```python
from build123d import *

# Parameters (mm, degrees)
ESQUISSE1_W             = 20
ESQUISSE1_H             = 52
BOSS_EXTRU_1_DEPTH      = 3
ESQUISSE2_R             = 1.5
ENL_V_MAT_EXTRU_1_DEPTH = 3
ESQUISSE3_R             = 5
ENL_V_MAT_EXTRU_2_DEPTH = 3
ESQUISSE4_W             = 3
ESQUISSE4_H             = 12
ENL_V_MAT_EXTRU_3_DEPTH = 10
ESQUISSE5_R             = 1
ENL_V_MAT_EXTRU_5_DEPTH = 10


with BuildPart() as part:
    # Esquisse1 → Boss.-Extru.1 (new body)
    with BuildSketch(Plane(origin=(0, 0, 0), x_dir=(1, 0, 0), z_dir=(0, 1, 0))):
        with Locations((-11.986036915, -31.933409069)):
            Rectangle(ESQUISSE1_W, ESQUISSE1_H)
    extrude(amount=BOSS_EXTRU_1_DEPTH)

    # Esquisse2 → Enlèv. mat.-Extru.1 (cut)
    with BuildSketch(Plane(origin=(0, 3, 0), x_dir=(1, 0, 0), z_dir=(0, 1, 0))):
        with Locations((-11.986036915, -41.933409069)):
            Circle(ESQUISSE2_R)
        with Locations((-11.986036915, -21.933409069)):
            Circle(ESQUISSE2_R)
    extrude(amount=-ENL_V_MAT_EXTRU_1_DEPTH, mode=Mode.SUBTRACT)

    # Esquisse3 → Enlèv. mat.-Extru.2 (cut)
    with BuildSketch(Plane(origin=(0, 3, 0), x_dir=(1, 0, 0), z_dir=(0, 1, 0))):
        with Locations((-23.986036915, -31.933409069)):
            Circle(ESQUISSE3_R)
    extrude(amount=-ENL_V_MAT_EXTRU_2_DEPTH, mode=Mode.SUBTRACT)

    # Esquisse4 → Enlèv. mat.-Extru.3 (cut)
    with BuildSketch(Plane(origin=(0, 3, 0), x_dir=(1, 0, 0), z_dir=(0, 1, 0))):
        with Locations((-13.486036915, -31.930984764)):
            Rectangle(ESQUISSE4_W, ESQUISSE4_H)
    extrude(amount=-ENL_V_MAT_EXTRU_3_DEPTH, mode=Mode.SUBTRACT)

    # Esquisse5 → Enlèv. mat.-Extru.5 (cut)
    with BuildSketch(Plane(origin=(0, 3, 0), x_dir=(1, 0, 0), z_dir=(0, 1, 0))):
        with Locations((-6.986036915, -35.330984764)):
            Circle(ESQUISSE5_R)
        with Locations((-6.986036915, -28.530984764)):
            Circle(ESQUISSE5_R)
    extrude(amount=-ENL_V_MAT_EXTRU_5_DEPTH, mode=Mode.SUBTRACT)


solid = part.part
```
Read the model definition and answer for the solid it produces. Units are mm, in the model's axes. A direction names the side the tool comes from. Coordinates: 2 decimals unless noted, no trailing zeros. Write each loop counter-clockwise with the first axis right and the second up, starting at its lowest first coordinate (ties: lowest second). Pieces come first, ordered by that corner, then holes. Notation, with made-up numbers: (49, -4) -> (89, -4) arc R32 ccw to (89, 23) -> close; hole circle Ø7 at (-27, 38.5). An arc over 180 degrees is marked (long way). Return JSON: item names as keys, results as strings.
1. A cutting plane is placed at B-B (y = 1.6). Determine the outline of the cut face in (x, z), and give its area (3 significant figures).
Found:
{"outline": "(-21.99, 5.93) -> (-1.99, 5.93) -> (-1.99, 57.93) -> (-21.99, 57.93) -> (-21.99, 36.52) arc R5 cw to (-21.99, 27.35) -> close; hole (-14.99, 25.93) -> (-11.99, 25.93) -> (-11.99, 37.93) -> (-14.99, 37.93) -> close; hole circle Ø3 at (-11.99, 21.93); hole circle Ø3 at (-11.99, 41.93); hole circle Ø2 at (-6.99, 28.53); hole circle Ø2 at (-6.99, 35.33)", "area": "964 mm2"}
2. A cutting plane is placed at C-C (z = 32.5). Determine the outline of the cut face in (x, y), and give its area (3 significant figures).
Found:
{"outline": "(-19.02, 0) -> (-14.99, 0) -> (-14.99, 3) -> (-19.02, 3) -> close; (-11.99, 0) -> (-1.99, 0) -> (-1.99, 3) -> (-11.99, 3) -> close", "area": "42.1 mm2"}
3. Each of these flat-tipped pins is pushed along its axis until it touches: P1, Ø3, axis at x = -7.5, z = 16, coming from the -Y side; P2, Ø1.5, axis at y = 2, z = 31, coming from the -X side. Where does it stop, or does it pass through?
Found:
{"P1": "y = 0", "P2": "x = -19.28"}
4. A tool of negligible diameter and unlimited length cuts with its end or side. For faces 4 (the face through (-14.986, 2, 32)), 5 (the face through (-10, 0, 32)), from which of +Z, -Z, +X, -X, +Y, -Y can it reach the whole face along a straight path? Write none if from no direction.
Found:
{"face 4": "+Y, -Y", "face 5": "+Z, -Z, +X, -X, -Y"}
5. Determine the mould class of faces 1 (the face through (-14, 2, 37.931)), 2 (the face through (-21.986, 1, 47)), 3 (the face through (-12, 1, 5.933)) for opening direction X: pulls with the +X half, pulls with the -X half, needs draft (parallel to the pull), parting line crosses it, or undercut.
Found:
{"face 1": "undercut", "face 2": "pulls with the -X half", "face 3": "needs draft"}
6. Find the intervals of material crossed by line 1 along Z through (x, y) = (-7, 2.3); line 2 along Z through (x, y) = (-14.5, 1.75); line 3 along Z through (x, y) = (-12.25, 0.45), in increasing order. Write a range as from..to.
Found:
{"line 1": "5.93..27.53, 29.53..34.33, 36.33..57.93", "line 2": "5.93..25.93, 37.93..57.93", "line 3": "5.93..20.46, 23.41..25.93, 37.93..40.46, 43.41..57.93"}
7. A cutting plane is placed at A-A (x = -20.5). Determine the outline of the cut face in (y, z).
Found:
{"outline": "(0, 5.93) -> (3, 5.93) -> (3, 28.35) -> (0, 28.35) -> close; (0, 35.52) -> (3, 35.52) -> (3, 57.93) -> (0, 57.93) -> close"}
